from build123d import *

# Parameters (mm, degrees)
SKETCH1_W           = 342.9
SKETCH1_H           = 342.9
BOSS_EXTRUDE1_DEPTH = 12.7
DRAFT1_ANGLE        = -45
SKETCH2_R           = 105.653774547
CUT_EXTRUDE1_DEPTH  = 243.799289538
CUT_EXTRUDE2_DEPTH  = 5.08


with BuildPart() as part:
    # Sketch1 → Boss-Extrude1 (new body)
    with BuildSketch(Plane.XY):
        Rectangle(SKETCH1_W, SKETCH1_H)
    extrude(amount=-BOSS_EXTRUDE1_DEPTH)

    # Draft1
    draft1_faces = [part.faces().sort_by_distance(p)[0] for p in [
        (-171.45, 0, -6.35),
        (0, -171.45, -6.35),
        (171.45, 0, -6.35),
        (0, 171.45, -6.35),
    ]]
    draft(draft1_faces, Plane.XY, DRAFT1_ANGLE)

    # Sketch2 → Cut-Extrude1 (cut, through all)
    with BuildSketch(Plane(origin=(0, 0, -12.7), x_dir=(-1, 0, 0), z_dir=(0, 0, -1))):
        Circle(SKETCH2_R)
    extrude(amount=-CUT_EXTRUDE1_DEPTH, mode=Mode.SUBTRACT)

    # Sketch3 → Cut-Extrude2 (cut)
    with BuildSketch(Plane(origin=(0, 0, -12.7), x_dir=(-1, 0, 0), z_dir=(0, 0, -1))):
        with BuildLine():
            Line((18.632943137, -145.166928512), (145.166928512, -18.632943137))
            ThreePointArc((145.166928512, -18.632943137), (154.686, -18.632943137), (154.686, -28.152014625))
            Line((154.686, -28.152014625), (28.152014625, -154.686))
            ThreePointArc((28.152014625, -154.686), (18.632943137, -154.686), (18.632943137, -145.166928512))
        make_face()
        with BuildLine():
            Line((-154.686, 28.152014625), (-28.152014625, 154.686))
            ThreePointArc((-28.152014625, 154.686), (-18.632943137, 154.686), (-18.632943137, 145.166928512))
            Line((-18.632943137, 145.166928512), (-145.166928512, 18.632943137))
            ThreePointArc((-145.166928512, 18.632943137), (-154.686, 18.632943137), (-154.686, 28.152014625))
        make_face()
    extrude(amount=-CUT_EXTRUDE2_DEPTH, mode=Mode.SUBTRACT)


solid = part.part
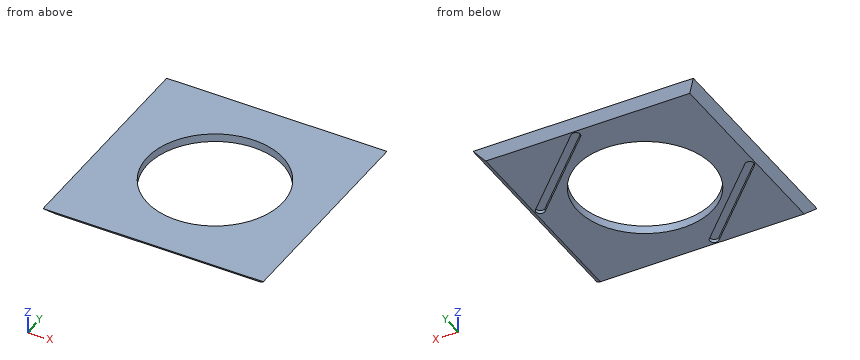
CAD build for the part. Positions are in the model's coordinates, mm. Round coordinates to 2 decimals unless told otherwise and drop trailing zeros. Order: outer loops, then holes, each group sorted by start corner. A loop starts at its lowest first (then second) coordinate and runs counter-clockwise, first axis right, second up. Notation, with made-up numbers: (51, 54.25) - (96, 54.25) arc R18 ccw to (96, 78.25) - close; hole circle Ø1 at (17, 17). An arc over 180 degrees is marked (long way). Return JSON: item names as keys, results as strings.
(1) Pin check, flat tips, straight feed: pin 1 Ø6 at (x, z) = (-11, -10.5) entering from -Y; pin 2 Ø3 at (x, z) = (-76, -10) entering from +Y; pin 3 Ø1.5 at (y, z) = (-74, -7) entering from +X. Stop position of each tip, or through.
Answer key:
{"pin 1": "stops at y = -163.95", "pin 2": "stops at y = 162.95", "pin 3": "stops at x = 165.2"}
(2) Wall check: probe 1 along Y at (x, z) = (-33, -9.5); probe 2 along Y at (x, z) = (72, -11.75); probe 3 along X at (y, z) = (-82, -11.25). Give the ranges that are in metal, low to high. Write a range as from..to.
Answer key:
{"probe 1": "y = -161.95..-149.84, -130.8..-100.37, 100.37..161.95", "probe 2": "y = -159.7..-77.32, 77.32..91.8, 110.84..159.7", "probe 3": "x = -160.2..-100.84, -81.8..-66.62, 66.62..160.2"}
(3) Cut at C-C (z = -10.5). Give the cut face in (x, y).
Answer key:
{"outline": "(-160.95, -160.95) - (160.95, -160.95) - (160.95, 160.95) - (-160.95, 160.95) - close; hole (-154.69, -28.15) - (-28.15, -154.69) arc R6.73 ccw to (-18.63, -145.17) - (-145.17, -18.63) arc R6.73 ccw to start; hole circle Ø211.31 at (0, 0); hole (18.63, 145.17) - (145.17, 18.63) arc R6.73 ccw to (154.69, 28.15) - (28.15, 154.69) arc R6.73 ccw to start"}
(4) Cut at D-D (x = 86). Give the cut face in (y, z), then the cut area to 3 significant figures.
Answer key:
{"outline": "(-171.45, 0) - (-158.75, -12.7) - (-61.37, -12.7) - (-61.37, 0) - close; (61.37, -12.7) - (77.8, -12.7) - (77.8, -7.62) - (96.84, -7.62) - (96.84, -12.7) - (158.75, -12.7) - (171.45, 0) - (61.37, 0) - close", "area": "2,540 mm^2"}
(5) Cut at A-A (x = 0). Give the cut face in (y, z), then the cut area to 3 significant figures.
Answer key:
{"outline": "(-171.45, 0) - (-158.75, -12.7) - (-105.65, -12.7) - (-105.65, 0) - close; (105.65, -12.7) - (158.75, -12.7) - (171.45, 0) - (105.65, 0) - close", "area": "1,510 mm^2"}
